The listing builds one solid part. Answer for the finished solid, in the listing's coordinates (mm). A direction names the side the tool comes from. Coordinates: 2 decimals unless noted, no trailing zeros. Loops run counter-clockwise (first coordinate to the right, second up) from the corner with the lowest first, then second, coordinate; pieces in that order, holes last. Notation, with made-up numbers: M 73.5,-23.5 L 101.5,-23.5 A19 cw 101.5,-4.5 Z; hole C 80.5,-32 d10. An arc over 180 degrees is marked long. Return JSON: item names as keys, results as strings. Group by question number.
1. Given P1, Ø1.5, axis at y = 1.5, z = -19.5, coming from the +X side, flat-ended and moving along its own axis, determine where the tip first touches the part or whether it passes through.
2. Section D-D (x = 26) is taken. Write down the section's boundary in (y, z).
3. The mould has two halves that part along Z. Classify faces 1 (the face through (24, 1.5, 21)), 2 (the face through (33.26, 1, 0)), 3 (the face through (23.382, 1.232, 23.655)): pulls with the +Z half, pulls with the -Z half, needs draft (parallel to the pull), parting line crosses it, or undercut.
4. Section B-B (y = 1.95) is taken. Count the separate pieces of the cut face and the enclosed holes in it, then the cut area to 3 significant figures.
5. Section A-A (x = 0) is taken. Write down the section's boundary in (y, z).
6. Section C-C (z = 11) is taken. Write down the section's boundary in (x, y).
7. Which of the six approach directions +Z, -Z, +X, -X, +Y, -Y give full straight-line access (tool end or side, diameter ignored) to faces 4 (the face through (10.18, 2.01, -10.07)), 5 (the face through (9, 2.5, 9)), 6 (the face through (0, 1, 12.32))?
8. Straight lines are drawn through the part: L1, parallel to Z at x = 5, y = 1.6; L2, parallel to Z at x = -19.5, y = 2; L3, parallel to X at y = 2.45, z = 20.5. For each, find the intervals that lie inside material, in ascending order. Write a range as from..to.
```python
from build123d import *

# Parameters (mm, degrees)
EXTRUDE_1_DEPTH     = 2.5
CUT_EXTRUDE_1_DEPTH = 1
CUT_EXTRUDE_2_DEPTH = 3.8
CUT_EXTRUDE_3_DEPTH = 1


with BuildPart() as part:
    # Sketch 1 → Extrude 1 (new body)
    with BuildSketch(Plane(origin=(0, 0, 0), x_dir=(1, 0, 0), z_dir=(0, 1, 0))):
        Polygon((-33.25966317, -13.776603565), (-13.776603565, -33.25966317), (13.776603565, -33.25966317), (33.25966317, -13.776603565), (33.25966317, 13.776603565), (13.776603565, 33.25966317), (-13.776603565, 33.25966317), (-33.25966317, 13.776603565), align=None)
        Polygon((-13.362390003, -32.25966317), (13.362390003, -32.25966317), (32.25966317, -13.362390003), (32.25966317, 13.362390003), (13.362390003, 32.25966317), (-13.362390003, 32.25966317), (-32.25966317, 13.362390003), (-32.25966317, -13.362390003), align=None, mode=Mode.SUBTRACT)
        Polygon((-32.25966317, -13.362390003), (-13.362390003, -32.25966317), (13.362390003, -32.25966317), (32.25966317, -13.362390003), (32.25966317, 13.362390003), (13.362390003, 32.25966317), (-13.362390003, 32.25966317), (-32.25966317, 13.362390003), align=None)
        Polygon((-12.94817644, -31.25966317), (12.94817644, -31.25966317), (31.25966317, -12.94817644), (31.25966317, 12.94817644), (12.94817644, 31.25966317), (-12.94817644, 31.25966317), (-31.25966317, 12.94817644), (-31.25966317, -12.94817644), align=None, mode=Mode.SUBTRACT)
        Polygon((-31.25966317, -12.94817644), (-12.94817644, -31.25966317), (12.94817644, -31.25966317), (31.25966317, -12.94817644), (31.25966317, 12.94817644), (12.94817644, 31.25966317), (-12.94817644, 31.25966317), (-31.25966317, 12.94817644), align=None)
    extrude(amount=EXTRUDE_1_DEPTH)

    # Sketch 2 → Cut-Extrude 1 (cut)
    with BuildSketch(Plane(origin=(0, 2.5, 0), x_dir=(1, 0, 0), z_dir=(0, 1, 0))):
        Polygon((13.279115103, -32.058619778), (32.058619778, -13.279115103), (32.058619778, 13.279115103), (13.279115103, 32.058619778), (-13.279115103, 32.058619778), (-32.058619778, 13.279115103), (-32.058619778, -13.279115103), (-13.279115103, -32.058619778), align=None)
        Polygon((12.864901541, -31.058619778), (31.058619778, -12.864901541), (31.058619778, 12.864901541), (12.864901541, 31.058619778), (-12.864901541, 31.058619778), (-31.058619778, 12.864901541), (-31.058619778, -12.864901541), (-12.864901541, -31.058619778), align=None, mode=Mode.SUBTRACT)
    extrude(amount=-CUT_EXTRUDE_1_DEPTH, mode=Mode.SUBTRACT)

    # Sketch 4 → Cut-Extrude 2 (cut)
    with BuildSketch(Plane(origin=(0, 2.5, 0), x_dir=(1, 0, 0), z_dir=(0, 1, 0))):
        Polygon((-12.320132754, -5.103166077), (-5.103166077, -12.320132754), (5.103166077, -12.320132754), (12.320132754, -5.103166077), (12.320132754, 5.103166077), (5.103166077, 12.320132754), (-5.103166077, 12.320132754), (-12.320132754, 5.103166077), align=None)
    extrude(amount=-CUT_EXTRUDE_2_DEPTH, mode=Mode.SUBTRACT)

    # Sketch 4_3 → Cut-Extrude 3 (cut)
    with BuildSketch(Plane(origin=(0, 2.5, 0), x_dir=(1, 0, 0), z_dir=(0, 1, 0))):
        Polygon((-14.320132754, -5.931593202), (-5.931593202, -14.320132754), (5.931593202, -14.320132754), (14.320132754, -5.931593202), (14.320132754, 5.931593202), (5.931593202, 14.320132754), (-5.931593202, 14.320132754), (-14.320132754, 5.931593202), align=None)
        Polygon((-5.517379639, -13.320132754), (5.517379639, -13.320132754), (13.320132754, -5.517379639), (13.320132754, 5.517379639), (5.517379639, 13.320132754), (-5.517379639, 13.320132754), (-13.320132754, 5.517379639), (-13.320132754, -5.517379639), align=None, mode=Mode.SUBTRACT)
    extrude(amount=-CUT_EXTRUDE_3_DEPTH, mode=Mode.SUBTRACT)


solid = part.part
```
Worked out:
{
 "1": {"P1": "x = 28.29"},
 "2": {"outline": "M 0,-21.04 L 2.5,-21.04 L 2.5,-19.34 L 1.5,-19.34 L 1.5,-17.92 L 2.5,-17.92 L 2.5,17.92 L 1.5,17.92 L 1.5,19.34 L 2.5,19.34 L 2.5,21.04 L 0,21.04 Z"},
 "3": {"face 1": "undercut", "face 2": "needs draft", "face 3": "pulls with the +Z half"},
 "4": {"separate pieces": "3", "enclosed holes": "3", "area": "2,860 mm^2"},
 "5": {"outline": "M 0,-33.26 L 2.5,-33.26 L 2.5,-32.06 L 1.5,-32.06 L 1.5,-31.06 L 2.5,-31.06 L 2.5,-14.32 L 1.5,-14.32 L 1.5,-13.32 L 2.5,-13.32 L 2.5,-12.32 L 0,-12.32 Z; M 0,12.32 L 2.5,12.32 L 2.5,13.32 L 1.5,13.32 L 1.5,14.32 L 2.5,14.32 L 2.5,31.06 L 1.5,31.06 L 1.5,32.06 L 2.5,32.06 L 2.5,33.26 L 0,33.26 Z"},
 "6": {"outline": "M -33.26,0 L -6.42,0 L -6.42,2.5 L -7.84,2.5 L -7.84,1.5 L -9.25,1.5 L -9.25,2.5 L -31.06,2.5 L -31.06,1.5 L -32.06,1.5 L -32.06,2.5 L -33.26,2.5 Z; M 6.42,0 L 33.26,0 L 33.26,2.5 L 32.06,2.5 L 32.06,1.5 L 31.06,1.5 L 31.06,2.5 L 9.25,2.5 L 9.25,1.5 L 7.84,1.5 L 7.84,2.5 L 6.42,2.5 Z"},
 "7": {"face 4": "+Y", "face 5": "+Z, -Z, +X, -X, +Y", "face 6": "+Y, -Y"},
 "8": {"L1": "-33.26..-32.06, -31.06..-14.32, -13.32..-12.32, 12.32..13.32, 14.32..31.06, 32.06..33.26", "L2": "-27.54..-25.84, -24.42..24.42, 25.84..27.54", "L3": "-26.54..-24.84, -23.42..23.42, 24.84..26.54"}
}
